Geometry check sheet. Reference: the model listing, model coordinates, mm. A direction names the side the tool comes from. Coordinates: 2 decimals unless noted, no trailing zeros. Write each loop counter-clockwise with the first axis right and the second up, starting at its lowest first coordinate (ties: lowest second). Pieces come first, ordered by that corner, then holes. Notation, with made-up numbers: (36, 52.5) -> (77, 52.5) arc R25 ccw to (77, 78.5) -> close; hole circle Ø3 at (18.5, 79.5). An arc over 180 degrees is marked (long way). Answer in a Markdown table with one row per item. Add a question column.
1. Cross-section at A-A on x = -21. Record the cut outline in (y, z).
2. Scan lines: L1, parallel to Y at x = -39, z = 0.8; L2, parallel to X at y = -98, z = 0.4; L3, parallel to Z at x = 19, y = 24. Record each from-to range of solid material in increasing order. Write a range as from..to.
3. Depth check by flat-ended pin: P1, Ø1.5, axis at y = -45.5, z = 3, coming from the +X side; P2, Ø5, axis at x = 12.5, z = 4.5, coming from the -Y side; P3, Ø2, axis at x = 24.5, z = -3, coming from the +Y side; P4, Ø1.3, axis at x = -39, y = 98, coming from the +Z side. Enter the tip coordinate at first touch or a pass-through.
4. Mould release check, pull along Y, two halves, no side actions. Record for faces 5 (the flat face through (0, 73, 4)), 6 (the flat face through (-12.5, -45, 4)), 7 (the flat face through (0, -92, 4)), 8 (the flat face through (0, -2, 4)): pulls with the +Y half, pulls with the -Y half, needs draft (parallel to the pull), parting line crosses it, or undercut.
5. Set-up check for faces 1 (the flat face through (12.5, 75, 4)), 2 (the flat face through (0, -7, -2)), 3 (the flat face through (0, -29, 6.588)), 4 (the flat face through (0, -47, 4)): record each of +Z, -Z, +X, -X, +Y, -Y from which the full face is reachable in a straight line by a thin tool's end or side.
6. Cross-section at B-B on y = -37. Record the cut outline in (x, z).
```python
from build123d import *

# Parameters (mm, degrees)
SKETCH1_W                 = 83
SKETCH1_H                 = 214
BOSS_EXTRUDE1_DEPTH       = 1.5875
SKETCH2_W                 = 25
SKETCH2_H                 = 5
BOSS_EXTRUDE2_DEPTH       = 5
F_0_CLEARANCE_HOLE1_D     = 1.6129
F_0_CLEARANCE_HOLE1_DEPTH = 3.175
F_0_CLEARANCE_HOLE1_TIP   = 0.484564046
SKETCH6_W                 = 72.5
SKETCH6_H                 = 7
BOSS_EXTRUDE3_DEPTH       = 4.9125


with BuildPart() as part:
    # Sketch1 → Boss-Extrude1 (new body)
    with BuildSketch(Plane.XY):
        Rectangle(SKETCH1_W, SKETCH1_H)
    extrude(amount=BOSS_EXTRUDE1_DEPTH)

    # Sketch2 → Boss-Extrude2 (add)
    with BuildSketch(Plane.XY.offset(1.5875)):
        with Locations((0, 90.5)):
            Rectangle(SKETCH2_W, SKETCH2_H)
        with Locations((0, 75.5)):
            Rectangle(SKETCH2_W, SKETCH2_H)
        with Locations((0, 60.5)):
            Rectangle(SKETCH2_W, SKETCH2_H)
        with Locations((0, 45.5)):
            Rectangle(SKETCH2_W, SKETCH2_H)
        with Locations((0, 30.5)):
            Rectangle(SKETCH2_W, SKETCH2_H)
        with Locations((0, 15.5)):
            Rectangle(SKETCH2_W, SKETCH2_H)
        with Locations((0, 0.5)):
            Rectangle(SKETCH2_W, SKETCH2_H)
        with Locations((0, -14.5)):
            Rectangle(SKETCH2_W, SKETCH2_H)
        with Locations((0, -29.5)):
            Rectangle(SKETCH2_W, SKETCH2_H)
        with Locations((0, -44.5)):
            Rectangle(SKETCH2_W, SKETCH2_H)
        with Locations((0, -59.5)):
            Rectangle(SKETCH2_W, SKETCH2_H)
        with Locations((0, -74.5)):
            Rectangle(SKETCH2_W, SKETCH2_H)
        with Locations((0, -89.5)):
            Rectangle(SKETCH2_W, SKETCH2_H)
    extrude(amount=BOSS_EXTRUDE2_DEPTH)

    # #0 Clearance Hole1
    with Locations(Plane.XY.offset(1.5875)):
        with Locations((-39, 98), (39, 98), (-39, 32.666666667), (39, 32.666666667), (-39, -32.666666667), (39, -32.666666667), (-39, -98), (39, -98)):
            Hole(F_0_CLEARANCE_HOLE1_D / 2, depth=F_0_CLEARANCE_HOLE1_DEPTH)
            with Locations((0, 0, -(F_0_CLEARANCE_HOLE1_DEPTH + F_0_CLEARANCE_HOLE1_TIP / 2))):  # 118° drill point
                Cone(0, F_0_CLEARANCE_HOLE1_D / 2, F_0_CLEARANCE_HOLE1_TIP, mode=Mode.SUBTRACT)

    # Sketch6 → Boss-Extrude3 (add)
    with BuildSketch(Plane(origin=(0, 0, 0), x_dir=(-1, 0, 0), z_dir=(0, 0, -1))):
        with Locations((0.05, -3.5)):
            Rectangle(SKETCH6_W, SKETCH6_H)
    extrude(amount=BOSS_EXTRUDE3_DEPTH)


solid = part.part
```
Results found:
| question | item | result |
|---|---|---|
| 1 | outline | (-107, 0) -> (-7, 0) -> (-7, -4.91) -> (0, -4.91) -> (0, 0) -> (107, 0) -> (107, 1.59) -> (-107, 1.59) -> close |
| 2 | L1 | y = -107..-98.81, -97.19..-33.47, -31.86..31.86, 33.47..97.19, 98.81..107 |
| 2 | L2 | x = -41.5..-39.81, -38.19..38.19, 39.81..41.5 |
| 2 | L3 | z = 0..1.59 |
| 3 | P1 | stops at x = 12.5 |
| 3 | P2 | stops at y = -92 |
| 3 | P3 | stops at y = 0 |
| 3 | P4 | passes through |
| 4 | face 5 | undercut |
| 4 | face 6 | needs draft |
| 4 | face 7 | pulls with the -Y half |
| 4 | face 8 | undercut |
| 5 | face 1 | +Z, +X, +Y, -Y |
| 5 | face 2 | -Z, +X, -X, -Y |
| 5 | face 3 | +Z, +X, -X, +Y, -Y |
| 5 | face 4 | +Z, +X, -X |
| 6 | outline | (-41.5, 0) -> (41.5, 0) -> (41.5, 1.59) -> (-41.5, 1.59) -> close |
